Input: part model. Units: mm. Frame: model coordinates. A direction names the side the tool comes from. Coordinates: 2 decimals unless noted, no trailing zeros. Loops run counter-clockwise (first coordinate to the right, second up) from the corner with the lowest first, then second, coordinate; pieces in that order, holes last. Notation, with made-up numbers: (57.25, -36.75) - (116.25, -36.75) arc R6 cw to (116.25, -32.75) - close; hole circle Ø8 at (17, 85). An arc over 180 degrees is marked (long way). Use one line per item in the form item = value.
from build123d import *

# Parameters (mm, degrees)
MODEL_W                = 13.999
MODEL_H                = 13.99947
MODEL_W_2              = 13.9993
MODEL_H_2              = 13.99948
MODEL_W_3              = 14.0009
MODEL_H_3              = 13.9994
MODEL_W_4              = 14
MODEL_W_5              = 13.9994
MODEL_H_4              = 13.9992
MODEL_W_6              = 13.9998
MODEL_W_7              = 13.99955
MODEL_W_8              = 14.0007
MODEL_W_9              = 14.001
MODEL_W_10             = 13.99954
MODEL_H_5              = 13.999
EXTRUDE_1_DEPTH        = 3
EXTRUDE_START          = -3
EXTRUDE_2_DEPTH        = 6
CUT_EXTRUDE_START      = -3
SKETCH_2_R             = 1.25
CUT_EXTRUDE_1_DEPTH    = 3.5
FILLET_1_R             = 1
PATTERN_LINEAR_1_COUNT = 3
PATTERN_LINEAR_1_PITCH = 90
SKETCH_3_R             = 1.25
CUT_EXTRUDE_2_DEPTH    = 3.5
PATTERN_LINEAR_2_COUNT = 3
PATTERN_LINEAR_2_PITCH = 70
CUT_EXTRUDE_3_DEPTH    = 10
FILLET_2_R             = 1


with BuildPart() as part:
    # Model → 凸台-拉伸1 (new body)
    with BuildSketch(Plane.XY):
        Polygon((4.85693, 129.021), (204.883, 129.021), (204.883, 0.434082), (14.38193, 0.434082), (14.38193, 24.241), (23.90693, 24.241), (23.90693, 43.291), (14.38193, 43.291), (14.38193, 62.341), (9.61893, 62.341), (9.61893, 81.391), (0.09393, 81.391), (0.09393, 109.971), (4.85693, 109.971), align=None)
        with Locations((152.4945, 9.959765)):
            Rectangle(MODEL_W, MODEL_H, mode=Mode.SUBTRACT)
        with Locations((171.5445, 9.959765)):
            Rectangle(MODEL_W, MODEL_H, mode=Mode.SUBTRACT)
        with Locations((190.5945, 9.959765)):
            Rectangle(MODEL_W, MODEL_H, mode=Mode.SUBTRACT)
        Polygon((33.5759, 21.722), (33.5759, 17.0215), (32.0504, 17.0215), (32.0504, 20.2517), (30.3251, 20.2517), (30.3251, 21.1722), (27.0261, 21.1722), (27.0261, 20.2517), (25.3008, 20.2517), (25.3008, 17.0215), (24.4753, 17.0215), (24.4753, 14.2227), (25.3008, 14.2227), (25.3008, 7.95267), (27.0261, 7.95267), (27.0261, 6.97286), (30.3251, 6.97286), (30.3251, 7.95267), (32.0504, 7.95267), (32.0504, 12.4216), (33.5759, 12.4216), (33.5759, 7.72252), (47.5753, 7.72252), (47.5753, 12.4216), (49.101, 12.4216), (49.101, 7.95267), (50.8247, 7.95267), (50.8247, 6.97286), (54.1253, 6.97286), (54.1253, 7.95267), (55.8504, 7.95267), (55.8504, 14.2227), (56.6759, 14.2227), (56.6759, 17.0215), (55.8504, 17.0215), (55.8504, 20.2517), (54.1253, 20.2517), (54.1253, 21.1722), (50.8247, 21.1722), (50.8247, 20.2517), (49.101, 20.2517), (49.101, 17.0215), (47.5753, 17.0215), (47.5753, 21.722), align=None, mode=Mode.SUBTRACT)
        with Locations((78.67565, 14.72226)):
            Rectangle(MODEL_W_2, MODEL_H_2, mode=Mode.SUBTRACT)
        with Locations((102.48755, 14.72226)):
            Rectangle(MODEL_W_3, MODEL_H_2, mode=Mode.SUBTRACT)
        with Locations((126.3005, 14.72226)):
            Rectangle(MODEL_W, MODEL_H_2, mode=Mode.SUBTRACT)
        with Locations((171.5445, 29.0097)):
            Rectangle(MODEL_W, MODEL_H_3, mode=Mode.SUBTRACT)
        with Locations((33.43185, 33.7722)):
            Rectangle(MODEL_W_2, MODEL_H_3, mode=Mode.SUBTRACT)
        with Locations((52.48185, 33.7722)):
            Rectangle(MODEL_W_2, MODEL_H_3, mode=Mode.SUBTRACT)
        with Locations((71.53185, 33.7722)):
            Rectangle(MODEL_W_2, MODEL_H_3, mode=Mode.SUBTRACT)
        with Locations((90.58185, 33.7722)):
            Rectangle(MODEL_W_2, MODEL_H_3, mode=Mode.SUBTRACT)
        with Locations((109.632, 33.7722)):
            Rectangle(MODEL_W_4, MODEL_H_3, mode=Mode.SUBTRACT)
        with Locations((135.8255, 33.7722)):
            Rectangle(MODEL_W, MODEL_H_3, mode=Mode.SUBTRACT)
        with Locations((195.357, 33.7722)):
            Rectangle(MODEL_W_4, MODEL_H_3, mode=Mode.SUBTRACT)
        Polygon((143.112, 59.8219), (143.112, 55.1215), (141.588, 55.1215), (141.588, 58.3516), (139.863, 58.3516), (139.863, 59.2723), (136.562, 59.2723), (136.562, 58.3516), (134.837, 58.3516), (134.837, 55.1215), (134.013, 55.1215), (134.013, 52.3226), (134.837, 52.3226), (134.837, 46.0527), (136.562, 46.0527), (136.562, 45.0716), (139.863, 45.0716), (139.863, 46.0527), (141.588, 46.0527), (141.588, 50.5217), (143.112, 50.5217), (143.112, 45.8227), (157.113, 45.8227), (157.113, 50.5217), (158.637, 50.5217), (158.637, 46.0527), (160.362, 46.0527), (160.362, 45.0716), (163.663, 45.0716), (163.663, 46.0527), (165.388, 46.0527), (165.388, 52.3226), (166.212, 52.3226), (166.212, 55.1215), (165.388, 55.1215), (165.388, 58.3516), (163.663, 58.3516), (163.663, 59.2723), (160.362, 59.2723), (160.362, 58.3516), (158.637, 58.3516), (158.637, 55.1215), (157.113, 55.1215), (157.113, 59.8219), align=None, mode=Mode.SUBTRACT)
        with Locations((23.9069, 52.8223)):
            Rectangle(MODEL_W_5, MODEL_H_4, mode=Mode.SUBTRACT)
        with Locations((42.95685, 52.8223)):
            Rectangle(MODEL_W_2, MODEL_H_4, mode=Mode.SUBTRACT)
        with Locations((62.00685, 52.8223)):
            Rectangle(MODEL_W_2, MODEL_H_4, mode=Mode.SUBTRACT)
        with Locations((81.05685, 52.8223)):
            Rectangle(MODEL_W_2, MODEL_H_4, mode=Mode.SUBTRACT)
        with Locations((100.1071, 52.8223)):
            Rectangle(MODEL_W_6, MODEL_H_4, mode=Mode.SUBTRACT)
        with Locations((119.157, 52.8223)):
            Rectangle(MODEL_W_4, MODEL_H_4, mode=Mode.SUBTRACT)
        with Locations((195.357, 52.8223)):
            Rectangle(MODEL_W_4, MODEL_H_4, mode=Mode.SUBTRACT)
        with Locations((19.1444, 71.8723)):
            Rectangle(MODEL_W_5, MODEL_H_4, mode=Mode.SUBTRACT)
        with Locations((38.19435, 71.8723)):
            Rectangle(MODEL_W_2, MODEL_H_4, mode=Mode.SUBTRACT)
        with Locations((57.24435, 71.8723)):
            Rectangle(MODEL_W_2, MODEL_H_4, mode=Mode.SUBTRACT)
        with Locations((76.29435, 71.8723)):
            Rectangle(MODEL_W_2, MODEL_H_4, mode=Mode.SUBTRACT)
        with Locations((95.34435, 71.8723)):
            Rectangle(MODEL_W_2, MODEL_H_4, mode=Mode.SUBTRACT)
        with Locations((114.3945, 71.8723)):
            Rectangle(MODEL_W, MODEL_H_4, mode=Mode.SUBTRACT)
        with Locations((133.4445, 71.8723)):
            Rectangle(MODEL_W, MODEL_H_4, mode=Mode.SUBTRACT)
        with Locations((157.257, 71.8723)):
            Rectangle(MODEL_W_4, MODEL_H_4, mode=Mode.SUBTRACT)
        with Locations((195.357, 71.8723)):
            Rectangle(MODEL_W_4, MODEL_H_4, mode=Mode.SUBTRACT)
        Polygon((145.493, 97.9219), (145.493, 93.2215), (143.969, 93.2215), (143.969, 96.4516), (142.244, 96.4516), (142.244, 97.3723), (138.943, 97.3723), (138.943, 96.4516), (137.218, 96.4516), (137.218, 93.2215), (136.394, 93.2215), (136.394, 90.4226), (137.218, 90.4226), (137.218, 84.1527), (138.943, 84.1527), (138.943, 83.1716), (142.244, 83.1716), (142.244, 84.1527), (143.969, 84.1527), (143.969, 88.6217), (145.493, 88.6217), (145.493, 83.9227), (159.494, 83.9227), (159.494, 88.6217), (161.018, 88.6217), (161.018, 84.1527), (162.743, 84.1527), (162.743, 83.1716), (166.044, 83.1716), (166.044, 84.1527), (167.768, 84.1527), (167.768, 90.4226), (168.593, 90.4226), (168.593, 93.2215), (167.768, 93.2215), (167.768, 96.4516), (166.044, 96.4516), (166.044, 97.3723), (162.743, 97.3723), (162.743, 96.4516), (161.018, 96.4516), (161.018, 93.2215), (159.494, 93.2215), (159.494, 97.9219), align=None, mode=Mode.SUBTRACT)
        with Locations((9.619425, 90.9223)):
            Rectangle(MODEL_W_7, MODEL_H_4, mode=Mode.SUBTRACT)
        with Locations((28.66935, 90.9223)):
            Rectangle(MODEL_W_2, MODEL_H_4, mode=Mode.SUBTRACT)
        with Locations((47.71935, 90.9223)):
            Rectangle(MODEL_W_2, MODEL_H_4, mode=Mode.SUBTRACT)
        with Locations((66.76935, 90.9223)):
            Rectangle(MODEL_W_2, MODEL_H_4, mode=Mode.SUBTRACT)
        with Locations((85.81935, 90.9223)):
            Rectangle(MODEL_W_2, MODEL_H_4, mode=Mode.SUBTRACT)
        with Locations((104.86865, 90.9223)):
            Rectangle(MODEL_W_8, MODEL_H_4, mode=Mode.SUBTRACT)
        with Locations((123.9185, 90.9223)):
            Rectangle(MODEL_W_9, MODEL_H_4, mode=Mode.SUBTRACT)
        with Locations((195.357, 90.9223)):
            Rectangle(MODEL_W_4, MODEL_H_4, mode=Mode.SUBTRACT)
        with Locations((14.38193, 119.4975)):
            Rectangle(MODEL_W_10, MODEL_H_5, mode=Mode.SUBTRACT)
        with Locations((33.43185, 119.4975)):
            Rectangle(MODEL_W_2, MODEL_H_5, mode=Mode.SUBTRACT)
        with Locations((52.48185, 119.4975)):
            Rectangle(MODEL_W_2, MODEL_H_5, mode=Mode.SUBTRACT)
        with Locations((71.53185, 119.4975)):
            Rectangle(MODEL_W_2, MODEL_H_5, mode=Mode.SUBTRACT)
        with Locations((90.58185, 119.4975)):
            Rectangle(MODEL_W_2, MODEL_H_5, mode=Mode.SUBTRACT)
        with Locations((109.632, 119.4975)):
            Rectangle(MODEL_W_4, MODEL_H_5, mode=Mode.SUBTRACT)
        with Locations((128.682, 119.4975)):
            Rectangle(MODEL_W_4, MODEL_H_5, mode=Mode.SUBTRACT)
        with Locations((152.4945, 119.4975)):
            Rectangle(MODEL_W, MODEL_H_5, mode=Mode.SUBTRACT)
        with Locations((171.5445, 119.4975)):
            Rectangle(MODEL_W, MODEL_H_5, mode=Mode.SUBTRACT)
        with Locations((192.9755, 119.4975)):
            Rectangle(MODEL_W, MODEL_H_5, mode=Mode.SUBTRACT)
    extrude(amount=EXTRUDE_1_DEPTH)

    # 草图1 → 凸台-拉伸2 (add)
    with BuildSketch(Plane.XY.offset(3).offset(EXTRUDE_START)):
        Polygon((14.38193, -4.565918), (209.883, -4.565918), (209.883, 134.021), (4.85693, 134.021), (4.85693, 129.021), (204.883, 129.021), (204.883, 0.434082), (14.38193, 0.434082), align=None)
    extrude(amount=EXTRUDE_2_DEPTH)

    # 草图2 → 切除-拉伸1 (cut)
    with BuildSketch(Plane.XY.offset(3).offset(CUT_EXTRUDE_START)):
        with Locations((7.85693, 131.521)):
            Circle(SKETCH_2_R)
        with Locations((17.38193, -2.065918)):
            Circle(SKETCH_2_R)
    cut_extrude_1 = extrude(amount=CUT_EXTRUDE_1_DEPTH, mode=Mode.SUBTRACT)

    # 圆角1
    fillet_1_edges = [part.edges().sort_by_distance(p)[0] for p in [
        (209.883, 134.021, 3),
        (4.85693, 134.021, 3),
        (14.38193, -4.565918, 3),
        (209.883, -4.565918, 3),
    ]]
    fillet(fillet_1_edges, radius=FILLET_1_R)

    # 阵列(线性)1: 切除-拉伸1 ×3
    with Locations(*[(i * PATTERN_LINEAR_1_PITCH, 0, 0) for i in range(1, PATTERN_LINEAR_1_COUNT)]):
        add(cut_extrude_1, mode=Mode.SUBTRACT)

    # 草图3 → 切除-拉伸2 (cut)
    with BuildSketch(Plane.XY.offset(3).offset(CUT_EXTRUDE_START)):
        with Locations((207.383, 35.434082)):
            Circle(SKETCH_3_R)
    cut_extrude_2 = extrude(amount=CUT_EXTRUDE_2_DEPTH, mode=Mode.SUBTRACT)

    # 阵列(线性)2: 切除-拉伸2 ×3
    with Locations(*[(0, i * PATTERN_LINEAR_2_PITCH, 0) for i in range(1, PATTERN_LINEAR_2_COUNT)]):
        add(cut_extrude_2, mode=Mode.SUBTRACT)

    # 草图4 → 切除-拉伸3 (cut)
    with BuildSketch(Plane.XY.offset(3)):
        Polygon((14.38193, 0.434082), (204.883, 0.434082), (204.883, 129.021), (4.85693, 129.021), (0.09393, 129.021), (0.09393, 0.434082), align=None)
    extrude(amount=-CUT_EXTRUDE_3_DEPTH, mode=Mode.SUBTRACT)

    # 圆角2
    fillet_2_edges = [part.edges().sort_by_distance(p)[0] for p in [
        (104.869965, 129.021, 6),
        (4.85693, 129.021, 3),
        (109.632465, 0.434082, 6),
        (204.883, 0.434082, 3),
        (204.883, 64.727541, 6),
        (204.883, 129.021, 3),
        (4.85693, 131.021, 6),
        (14.38193, 0.434082, 3),
        (112.132465, -4.565918, 6),
        (14.38193, -1.565918, 6),
        (107.369965, 134.021, 6),
        (209.883, 64.727541, 6),
        (209.590106781, -4.273024781, 6),
        (209.590106781, 133.728106781, 6),
        (5.149823219, 133.728106781, 6),
        (14.674823219, -4.273024781, 6),
    ]]
    fillet(fillet_2_edges, radius=FILLET_2_R)


solid = part.part
Q1. Cut plane A-A, the plane x = 183.5. Return loops of the section in (y, z).
Check values:
outline = (-4.57, 0) - (0.43, 0) - (0.43, 5) arc R1 ccw to (-0.57, 6) - (-3.57, 6) arc R1 ccw to (-4.57, 5) - close; (129.02, 0) - (134.02, 0) - (134.02, 5) arc R1 ccw to (133.02, 6) - (130.02, 6) arc R1 ccw to (129.02, 5) - close
Q2. Ray query, line 1 along Y through (x, z) = (189, 5.2); line 2 along Y through (x, z) = (196, 3.5); line 3 along X through (y, z) = (79, 4.6). Return the intervals inside material, ascending. Write a range as [from, to].
Check values:
line_1 = [-4.55, 0.41], [129.04, 134]
line_2 = [-4.57, 0.43], [129.02, 134.02]
line_3 = [204.88, 209.88]
Q3. First-contact query: P1, Ø2, axis at y = 117.5, z = 1.5, coming from the -X side; P2, Ø1.5, axis at y = -2, z = 2.5, coming from the -X side; P3, Ø0.8, axis at x = 207, y = 35, coming from the -Z side; P4, Ø3, axis at x = 18, y = -2, coming from the -Z side. Flat tips, straight axial feed; report the tip coordinate or a pass-through.
Check values:
P1 = 204.88
P2 = 14.38
P3 = 3.5
P4 = 0
Q4. Set-up query: faces 1 (the flat face through (108, 0.434, 3)), 2 (the flat face through (206, 65, 0)). Return all of +Z, -Z, +X, -X, +Y, -Y with unobstructed straight access to the full face (end or side cutting, diameter ignored); none if empty.
Check values:
face_1 = +Z, -Z, -X
face_2 = -Z, +X, -X, +Y, -Y
Q5. Cut plane C-C, the plane y = 23. Return loops of the section in (x, z), then the cut area to 3 significant figures.
Check values:
outline = (204.88, 0) - (209.88, 0) - (209.88, 5) arc R1 ccw to (208.88, 6) - (205.88, 6) arc R1 ccw to (204.88, 5) - close
area = 29.6 mm²
Q6. Cut plane B-B, the plane z = 1.3. Give the number of separate pieces and of enclosed holes in the cut face, then the cut area to 3 significant figures.
Check values:
separate_pieces = 1
enclosed_holes = 8
area = 2,610 mm²
